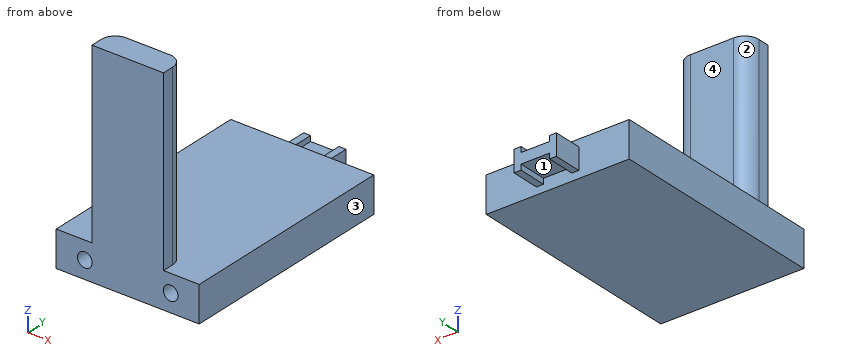
```python
from build123d import *

# Parameters (mm, degrees)
SKETCH3_W           = 101.6
SKETCH3_H           = 25.4
BOSS_EXTRUDE1_DEPTH = 157.8
BOSS_EXTRUDE4_DEPTH = 20.32
SKETCH7_R           = 5.207
CUT_EXTRUDE1_DEPTH  = 17.78
SKETCH8_W           = 50.8
SKETCH8_H           = 18.321584398
BOSS_EXTRUDE5_DEPTH = 127
FILLET1_R           = 10
FILLET2_R           = 10


with BuildPart() as part:
    # Sketch3 → Boss-Extrude1 (new body)
    with BuildSketch(Plane(origin=(0, 0, 0), x_dir=(1, 0, 0), z_dir=(0, 1, 0))):
        with Locations((25.4, 12.7)):
            Rectangle(SKETCH3_W, SKETCH3_H)
    extrude(amount=BOSS_EXTRUDE1_DEPTH)

    # Sketch6 → Boss-Extrude4 (add)
    with BuildSketch(Plane(origin=(0, 157.8, 0), x_dir=(1, 0, 0), z_dir=(0, 1, 0))):
        Polygon((10.447692892, 20.189678665), (15.293534065, 20.189678665), (15.293534065, 16.409589502), (35.527040487, 16.409589502), (35.527040487, 20.263619063), (40.533430612, 20.263619063), (40.533430612, 5.114574025), (35.460110097, 5.114574025), (35.460110097, 8.942217594), (15.367197577, 8.942217594), (15.367197577, 5.087318386), (10.388766814, 5.087318386), align=None)
    extrude(amount=BOSS_EXTRUDE4_DEPTH)

    # Sketch7 → Cut-Extrude1 (cut)
    with BuildSketch(Plane(origin=(0, 0, 0), x_dir=(-1, 0, 0), z_dir=(0, -1, 0))):
        with Locations(Location((5.08, 12.7, 0), (0, 0, 90))):
            Circle(SKETCH7_R)
        with Locations(Location((-55.88, 12.7, 0), (0, 0, 90))):
            Circle(SKETCH7_R)
    extrude(amount=-CUT_EXTRUDE1_DEPTH, mode=Mode.SUBTRACT)

    # Sketch8 → Boss-Extrude5 (add)
    with BuildSketch(Plane.XY):
        with Locations((25.4, 9.160792199)):
            Rectangle(SKETCH8_W, SKETCH8_H)
    extrude(amount=BOSS_EXTRUDE5_DEPTH)

    # Fillet1
    fillet1_edges = [part.edges().sort_by_distance(p)[0] for p in [
        (50.8, 18.321584398, 63.5),
    ]]
    fillet(fillet1_edges, radius=FILLET1_R)

    # Fillet2
    fillet2_edges = [part.edges().sort_by_distance(p)[0] for p in [
        (0, 18.321584398, 63.5),
    ]]
    fillet(fillet2_edges, radius=FILLET2_R)


solid = part.part
```
Here's how the part is built. I have some questions about the finished solid (model axes, mm). Face numbers are marked on the shaded views. A direction names the side the tool comes from. Give positions to 0.01 mm unless a question says otherwise; leave off trailing zeros. Loops run counter-clockwise (first coordinate to the right, second up) from the corner with the lowest first, then second, coordinate; pieces in that order, holes last. Notation, with made-up numbers: M 65.25,-17 L 80.25,-17 A31 cw 80.25,20 Z; hole C 59.25,55.25 d10. An arc over 180 degrees is marked long. Put each result on its own line as item: value. Start each with the question number.
(1) I want a section at D-D on z = -12.7. Please give me the cut outline in (x, y), then the cut area to 3 significant figures.
(2) I want a section at B-B on y = 76. Please give me the cut outline in (x, z).
(3) I want a section at A-A on x = 55.88. Please give me the cut outline in (y, z), then the cut area to 3 significant figures.
(4) I want a section at C-C on z = 52. Please give me the cut outline in (x, y), then the cut area to 3 significant figures.
(5) Will these pins go through, and if not, where does the flat tip stop? pin 1 Ø9 at (x, z) = (27, 92) entering from +Y; pin 2 Ø1.5 at (x, y) = (12, 170) entering from -Z; pin 3 Ø9.5 at (x, z) = (55.88, -12.7) entering from -Y.
(6) For the marked faces 1, 2, 3 and 4, which set-ups out of +Z, -Z, +X, -X, +Y, -Y let a thin tool reach every point of the face, with its end or its side?
(7) I need wall thicknesses on line 1 along X through (y, z) = (5, -12); line 2 along X through (y, z) = (4.75, -12.7); line 3 along Z through (x, y) = (10, 36). Which ranges of each line are inside material? Lowest first, please. Write a range as [from, to].
Answer block:
1. outline: M -25.4,0 L -10.29,0 L -10.29,17.78 L 0.13,17.78 L 0.13,0 L 50.67,0 L 50.67,17.78 L 61.09,17.78 L 61.09,0 L 76.2,0 L 76.2,157.8 L 40.53,157.8 L 40.53,178.12 L 10.42,178.12 L 10.42,157.8 L -25.4,157.8 Z
1. area: 16,300 mm^2
2. outline: M -25.4,-25.4 L 76.2,-25.4 L 76.2,0 L -25.4,0 Z
3. outline: M 0,-25.4 L 157.8,-25.4 L 157.8,0 L 0,0 L 0,-7.49 L 17.78,-7.49 L 17.78,-17.91 L 0,-17.91 Z
3. area: 3,820 mm^2
4. outline: M 0,0 L 50.8,0 L 50.8,8.32 A10 ccw 40.8,18.32 L 10,18.32 A10 ccw 0,8.32 Z
4. area: 888 mm^2
5. pin 1: y = 18.32
5. pin 2: z = -20.19
5. pin 3: y = 17.78
6. face 1: -Z, +Y
6. face 2: +Z, -X, +Y
6. face 3: +Z, -Z, +X, +Y, -Y
6. face 4: +Z, +X, -X, +Y
7. line 1: [-25.4, -10.24], [0.08, 50.72], [61.04, 76.2]
7. line 2: [-25.4, -10.29], [0.13, 50.67], [61.09, 76.2]
7. line 3: [-25.4, 0]
